Build history of the part. All positions in model axes, mm. A direction names the side the tool comes from. Round coordinates to 2 decimals unless told otherwise and drop trailing zeros. Write each loop counter-clockwise with the first axis right and the second up, starting at its lowest first coordinate (ties: lowest second). Pieces come first, ordered by that corner, then holes. Notation, with made-up numbers: (-2.5, -38.5) - (46.5, -38.5) arc R19 ccw to (46.5, -28.5) - close; hole circle Ø2 at (32, 65.25). An arc over 180 degrees is marked (long way). Answer as a JSON object with one key per item and string values. Group by question number.
Item 1: Slice it at C-C, the plane y = 1.25. List the corners of the cut face in (x, z) (3 decimals), then the cut area to 3 significant figures.
Item 2: Two-plate mould, pull along Z, no slides. Class faces 1 (the flat face through (-24, 0, 12)), 2 (the cylindrical face through (-24.653, 0.373, -2.445)), 3 (the cylindrical face through (-24.688, 3.18, -1.813)): +Z half, -Z half, draft (parallel to the pull), parting line (faces both ways), or undercut.
Item 3: Slice it at D-D, the plane x = -23.1. List the corners of the cut face in (y, z) (3 decimals).
Item 4: Slice it at A-A, the plane y = 3.5. List the corners of the cut face in (x, z) (3 decimals), then the cut area to 3 significant figures.
Item 5: Probe line 1 (X direction, y = 2, z = 26); line 2 (Z direction, x = -23.65, y = 3.75) (3 decimals); line 3 (X direction, y = 4.75, z = 7). List the from-to ranges inside material, lowest first. Write a range as from..to.
Item 6: Which spindle directions (+Z, -Z, +X, -X, +Y, -Y) get a long thin tool onto all of the face, cutting with end or side? Do faces 4 (the flat face through (-23.4, 3, 2)), 5 (the flat face through (-24.015, 3, 23)), 6 (the flat face through (-21.475, 3, 23)). Say none if no direction does.
Item 7: Flat gauge pins, fed straight in: pin 1 (2 mm diameter, centred on x = -24.5, y = 4.5, fed in from +Z); pin 2 (2.5 mm diameter, centred on y = 3.13, z = -0.77, fed in from +X); pin 3 (1.5 mm diameter, centred on x = -24, z = 7, fed in from -Y). Where does each tip first touch, or does it go through?
Item 8: Slice it at B-B, the plane x = -25.2. List the corners of the cut face in (y, z) (3 decimals), then the cut area to 3 significant figures.
from build123d import *

# Parameters (mm, degrees)
BOSS_EXTRUDE1_DEPTH     = 6.35
CUT_EXTRUDE1_DEPTH      = 30.397829873
CUT_EXTRUDE1_DEPTH_BACK = 3.556
CUT_EXTRUDE2_START      = -2.54
CUT_EXTRUDE2_DEPTH      = 2.54
SKETCH4_3_R             = 1.0414
CUT_EXTRUDE3_DEPTH      = 2.54
SKETCH3_3_R             = 1.0414
CUT_EXTRUDE4_DEPTH      = 2.54


# Read off the part's stored shape, not the designer's step: Cut-Extrude2
with BuildPart() as part:
    # Sketch1 → Boss-Extrude1 (new body)
    with BuildSketch(Plane(origin=(0, 0, 0), x_dir=(1, 0, 0), z_dir=(0, 1, 0))):
        Polygon((-24.015298923, -26.283339213), (-24.015298923, -25.179419289), (-24.015298923, -17.460268456), (-25.940364211, -7.62), (-25.940364211, 3.175), (-23.400364211, 3.175), (-23.400364211, -7.62), (-21.475298923, -17.460268456), (-21.475298923, -25.179419289), (-21.475298923, -28.354419289), (-24.015298923, -28.354419289), align=None)
    extrude(amount=BOSS_EXTRUDE1_DEPTH)

    # Sketch3 → Cut-Extrude1 (cut, two sides: drawn at the far end of the back side and taken through both)
    with BuildSketch(Plane.ZY.offset(25.940364211).offset(-CUT_EXTRUDE1_DEPTH_BACK)):
        with BuildLine():
            Line((68.316456583, 0.312090818), (-0.490666477, 6.35))
            ThreePointArc((-0.490666477, 6.35), (-3.991378408, 2.885541924), (0, 0))
            Line((0, 0), (67.062782235, 16.536619059))
            Line((67.062782235, 16.536619059), (-70.669713894, 5.893986208))
            Line((-70.669713894, 5.893986208), (-69.416039547, -10.330542032))
            Line((-69.416039547, -10.330542032), (68.316456583, 0.312090818))
        make_face()
    extrude(amount=CUT_EXTRUDE1_DEPTH + CUT_EXTRUDE1_DEPTH_BACK, mode=Mode.SUBTRACT)


with BuildPart() as cut_extrude1_kept_piece:
    # of the separate pieces the step leaves, the one the design keeps (cut_extrude1_pieces_kept)
    add(part.part.solids().sort_by_distance((-24.015298923, 0, 17.460268456))[0])

    # Cut-Extrude2 outline → Cut-Extrude2 (cut)
    with BuildSketch(Plane.ZY.offset(24.015298923).offset(CUT_EXTRUDE2_START)):
        with BuildLine():
            Line((28.354419289, 6.35), (25.179419289, 6.35))
            ThreePointArc((25.179419289, 6.35), (27.424483319, 5.42006403), (28.354419289, 3.175))
            Line((28.354419289, 3.175), (28.354419289, 6.35))
        make_face()
        with BuildLine():
            Line((28.354419289, 0), (28.354419289, 3.175))
            ThreePointArc((28.354419289, 3.175), (27.424483319, 0.92993597), (25.179419289, 0))
            Line((25.179419289, 0), (28.354419289, 0))
        make_face()
    extrude(amount=CUT_EXTRUDE2_DEPTH, mode=Mode.SUBTRACT)

    # Sketch4<3> → Cut-Extrude3 (cut)
    with BuildSketch(Plane.ZY.offset(24.015298923)):
        with Locations((25.179419289, 3.175)):
            Circle(SKETCH4_3_R)
    extrude(amount=-CUT_EXTRUDE3_DEPTH, mode=Mode.SUBTRACT)

    # Sketch3<3> → Cut-Extrude4 (cut)
    with BuildSketch(Plane.ZY.offset(25.940364211)):
        with Locations((-0.772853494, 3.134238346)):
            Circle(SKETCH3_3_R)
    extrude(amount=-CUT_EXTRUDE4_DEPTH, mode=Mode.SUBTRACT)


solid = cut_extrude1_kept_piece.part
Geometry says:
{
 "1": {"outline": "(-25.94, -3.175) - (-23.4, -3.175) - (-23.4, 7.62) - (-21.475, 17.46) - (-21.475, 27.704) - (-24.015, 27.704) - (-24.015, 17.46) - (-25.94, 7.62) - close", "area": "78.4 mm^2"},
 "2": {"face 1": "draft", "face 2": "-Z half", "face 3": "undercut"},
 "3": {"outline": "(0, 9.155) - (6.35, 9.155) - (6.35, 25.179) arc R3.175 ccw to (0, 25.179) - close; hole circle Ø2.083 at (3.175, 25.179)"},
 "4": {"outline": "(-25.94, -3.175) - (-23.4, -3.175) - (-23.4, -1.748) - (-25.94, -1.748) - close; (-25.94, 0.202) - (-23.4, 0.202) - (-23.4, 7.62) - (-21.475, 17.46) - (-21.475, 24.19) - (-24.015, 24.19) - (-24.015, 17.46) - (-25.94, 7.62) - close; (-24.015, 26.169) - (-21.475, 26.169) - (-21.475, 28.338) - (-24.015, 28.338) - close", "area": "70.1 mm^2"},
 "5": {"line 1": "x = -24.02..-21.48", "line 2": "z = -3.175..-1.613, 0.067..24.311, 26.048..28.302", "line 3": "x = -25.94..-23.4"},
 "6": {"face 4": "-Z, +X, +Y, -Y", "face 5": "+Z, -X, +Y, -Y", "face 6": "+Z, -Z, +X, +Y, -Y"},
 "7": {"pin 1": "stops at z = 28.32", "pin 2": "stops at x = -23.4", "pin 3": "stops at y = 0"},
 "8": {"outline": "(0, -1.546) arc R3.228 ccw to (0.978, -3.175) - (5.291, -3.175) arc R3.228 ccw to (6.35, -1.055) - (6.35, 11.404) - (0, 11.404) - close; hole circle Ø2.083 at (3.134, -0.773)", "area": "87.8 mm^2"}
}
